For this review, take the finished solid that the model builds, in its own axes (mm). A direction names the side the tool comes from. Round coordinates to 2 decimals unless told otherwise and drop trailing zeros. Write each loop counter-clockwise with the first axis right and the second up, starting at its lowest first coordinate (ties: lowest second). Pieces come first, ordered by that corner, then holes. Notation, with made-up numbers: (18.5, 34) - (58.5, 34) arc R28 ccw to (58.5, 58) - close; hole circle Ø2 at (52, 87.25). An arc over 180 degrees is marked (long way). Answer in a Markdown table with one row per item. Add a question column.
from build123d import *

# Parameters (mm, degrees)
F1_DEPTH = 4.5
F3_DEPTH = 6
F5_DEPTH = 4.5
F7_DEPTH = 3.001
F8_R     = 1.5
F9_DEPTH = 25


with BuildPart() as f1:
    # F0 (on Front) → F1 (new body)
    with BuildSketch(Plane.XZ):
        Polygon((0, 20), (0, 0), (20, 0), align=None)
    extrude(amount=F1_DEPTH)

    # F2 (on face) → F3 (join)
    with BuildSketch(Plane.XZ.offset(4.5)):
        Polygon((15, 3), (3, 3), (3, 15), (3, 17), (0, 20), (0, 0), (20, 0), (17, 3), align=None)
    extrude(amount=F3_DEPTH)

    # F4 (on face) → F5 (join)
    with BuildSketch(Plane.XZ.offset(10.5)):
        Polygon((20, 0), (0, 20), (0, 0), align=None)
    extrude(amount=F5_DEPTH)

    # F6 (on face) → F7 (cut, through all)
    with BuildSketch(Plane.YZ.offset(3)):
        with BuildLine():
            ThreePointArc((-7.5, 15.5), (-8.56066, 12.93934), (-6, 14))
            ThreePointArc((-6, 14), (-6.43934, 15.06066), (-7.5, 15.5))
        make_face()
    extrude(amount=-F7_DEPTH, mode=Mode.SUBTRACT)

    # F8 (on face) → F9 (cut)
    with BuildSketch(Plane.XY.offset(3)):
        with Locations((14, -7.5)):
            Circle(F8_R)
    extrude(amount=-F9_DEPTH, mode=Mode.SUBTRACT)


solid = f1.part
Q1. Draft analysis for pull direction Y (two halves, no side actions). For faces 1 (the face through (10, -4, 10)), 2 (the face through (7, -10.5, 7)), 3 (the face through (5, -15, 6)), state which applies: released by +Y, released by -Y, zero draft, split by the parting line, or undercut.
Q2. To check wall thickness, follow probe 1 along Y at (x, z) = (0.8, 14); probe 2 along Y at (x, z) = (6.5, 10.5); probe 3 along X at (y, z) = (-1, 3). State the ranges of each line that lie inside material, in increasing order.
Q3. Add section A-A on x = 14. State the section outline as (y, z) points, then the cut area to 3 significant figures.
Q4. Add section D-D on x = 10.5. State the section outline as (y, z) points.
Q5. Add section B-B on y = -8. State the section outline as (x, z) points, then the cut area to 3 significant figures.
Q6. Add section C-C on z = 1.5. State the section outline as (x, y) points.
Q7. Tool access review of faces 4 (the face through (5, 0, 6)), 5 (the face through (3, -7, 10)): name each direction out of +Z, -Z, +X, -X, +Y, -Y from which nothing blocks a thin tool from reaching the whole face with its end or side.
Q8. Insertion check: pin 1 Ø3 at (y, z) = (-3.5, 16) entering from +X; pin 2 Ø4 at (x, y) = (11, -13.5) entering from +Z; pin 3 Ø2 at (x, y) = (16, -4) entering from +Z. Each pin has a flat end and moves straight along its axis. Give the tip position at first contact, or say it passes through.
Answer sheet:
| question | item | result |
|---|---|---|
| 1 | face 1 | zero draft |
| 1 | face 2 | undercut |
| 1 | face 3 | released by -Y |
| 2 | probe 1 | y = -15 to -9, -6 to 0 |
| 2 | probe 2 | y = -15 to -10.5, -4.5 to 0 |
| 2 | probe 3 | x = 0 to 17 |
| 3 | outline | (-15, 0) - (-9, 0) - (-9, 3) - (-10.5, 3) - (-10.5, 6) - (-15, 6) - close; (-6, 0) - (0, 0) - (0, 6) - (-4.5, 6) - (-4.5, 3) - (-6, 3) - close |
| 3 | area | 63.0 mm² |
| 4 | outline | (-15, 0) - (0, 0) - (0, 9.5) - (-4.5, 9.5) - (-4.5, 3) - (-10.5, 3) - (-10.5, 9.5) - (-15, 9.5) - close |
| 5 | outline | (0, 0) - (12.59, 0) - (12.59, 3) - (3, 3) - (3, 12.59) - (0, 12.59) - close; (0, 15.41) - (3, 15.41) - (3, 17) - (0, 20) - close; (15.41, 0) - (20, 0) - (17, 3) - (15.41, 3) - close |
| 5 | area | 85.0 mm² |
| 6 | outline | (0, -15) - (18.5, -15) - (18.5, 0) - (0, 0) - close; hole circle Ø3 at (14, -7.5) |
| 7 | face 4 | +Z, -Z, +X, -X, +Y |
| 7 | face 5 | +Z, +X |
| 8 | pin 1 | stops at x = 5.5 |
| 8 | pin 2 | stops at z = 11 |
| 8 | pin 3 | stops at z = 5 |
